Geometry check sheet. Reference: the model listing, model coordinates, mm. Give positions to 0.01 mm unless a question says otherwise; leave off trailing zeros. Write item = value, one per line. Start each with the question number.
1. Mould release check, pull along Y, two halves, no side actions. Record for faces 1 (the flat face through (0, -952.5, 1)), 2 (the flat face through (0, -13, -44.45)), 3 (the flat face through (0, 952.5, 1)): pulls with the +Y half, pulls with the -Y half, needs draft (parallel to the pull), parting line crosses it, or undercut.
2. Thickness scan on line 1 along Z through (x, y) = (11, -933.45); line 2 along Z through (x, y) = (-17, 30). Record the ranges inside material, lowest first.
3. Depth check by flat-ended pin: P1, Ø4, axis at y = 933.45, z = -22.225, coming from the +X side. Enter the tip coordinate at first touch or a pass-through.
```python
from build123d import *

# Parameters (mm, degrees)
F0_W          = 38.1
F0_H          = 88.9
F1_DEPTH      = 952.5
F1_DEPTH_BACK = 952.5
F2_R          = 3.175
F3_DEPTH      = 12.7
F4_R          = 2.54


# Not quite as in the source:
# - a length typed as a fraction of an inch, garbled in the dataset ("3 / 203.2 mm" for 3/8 in), is restored
# - a pattern or mirror of a feature is missing from the dataset's text; its kind, count and spacing are read off the source's solid


with BuildPart() as f1:
    # F0 (on Front) → F1 (new body, two sides)
    with BuildSketch(Plane.XZ) as f1_sk:
        Rectangle(F0_W, F0_H)
    extrude(amount=F1_DEPTH)
    extrude(f1_sk.sketch, amount=-F1_DEPTH_BACK)

    # F2 (on face) → F3 (cut)
    with BuildSketch(Plane.YZ.offset(19.05)):
        with Locations((-933.45, 22.225)):
            Circle(F2_R)
    f3 = extrude(amount=-F3_DEPTH, mode=Mode.SUBTRACT)

    # F3_copies: F3 across plane
    add(f3.mirror(Plane(origin=(0, 0, 0), x_dir=(0, 0.0238027779, 0.9997166737), z_dir=(0, 0.9997166737, -0.0238027779))), mode=Mode.SUBTRACT)

    # F3_copies1: F3 across plane
    add(f3.mirror(Plane(origin=(0, 0, 0), x_dir=(-1, 0, 0), z_dir=(0, 0, -1))), mode=Mode.SUBTRACT)

    # F3_copies2: F3 across plane
    add(f3.mirror(Plane.ZX), mode=Mode.SUBTRACT)

    # F4
    f4_edges = [f1.edges().sort_by_distance(p)[0] for p in [
        (19.05, 0, 44.45),
        (-19.05, 0, 44.45),
        (19.05, 0, -44.45),
        (-19.05, 0, -44.45),
    ]]
    fillet(f4_edges, radius=F4_R)


solid = f1.part
```
Answers:
q1.face_1 = pulls with the -Y half
q1.face_2 = needs draft
q1.face_3 = pulls with the +Y half
q2.line_1 = -44.45 to -25.4, -19.05 to 19.05, 25.4 to 44.45
q2.line_2 = -44.4 to 44.4
q3.P1 = 6.35
